Autodesk Inventor part; units mm, degrees
ref_plane "YZ Plane" through (0, 0, 0) normal (1, 0, 0) x (0, 1, 0)
ref_plane "XZ Plane" through (0, 0, 0) normal (0, 1, 0) x (-1, 0, 0)
ref_plane "XY Plane" through (0, 0, 0) normal (0, 0, 1) x (1, 0, 0)
sketch "Sketch1" plane through (0, 0, 0) normal (0, 0, 1) x (1, 0, 0)
  line L0 (-185.0798, 623.3432) -> (284.8202, 623.3432)
  line L1 (284.8202, 623.3432) -> (284.8202, -278.3568)
  line L2 (284.8202, -278.3568) -> (-185.0798, -278.3568)
  line L3 (-185.0798, -278.3568) -> (-185.0798, 623.3432)
  point P0 (0, 0)
  dimension "d0" = 901.7
  dimension "d1" = 469.9
extrude "Board" add sketch "Sketch1" along normal blind 19.05
sketch "Sketch6" plane through (0, 0, 0) normal (0, 0, -1) x (-1, 0, 0)
  line L0 (-284.8202, 483.6432) -> (185.0798, 483.6432)
  line L1 (185.0798, 483.6432) -> (185.0798, 464.5932)
  line L2 (185.0798, 464.5932) -> (-284.8202, 464.5932)
  line L3 (-284.8202, 464.5932) -> (-284.8202, 483.6432)
  line L4 (185.0798, 623.3432) -> (-284.8202, 623.3432)
  line L5 (185.0798, -278.3568) -> (185.0798, 623.3432)
  line L6 (-284.8202, 623.3432) -> (-284.8202, -278.3568)
  line L7 (-284.8202, 29.6182) -> (185.0798, 29.6182)
  line L8 (185.0798, 29.6182) -> (185.0798, 10.5682)
  line L9 (185.0798, 10.5682) -> (-284.8202, 10.5682)
  line L10 (-284.8202, 10.5682) -> (-284.8202, 29.6182)
  point P0 (0, 0)
  dimension "d30" = 19.05
  dimension "d37" = 434.975
  dimension "d119" = 139.7
extrude "Right Shelf Dados" cut sketch "Sketch6" against normal blind 6.35 contours L0 L1 L2 L3 | L7 L5 L9 L6
sketch "Sketch32" plane through (0, 0, 0) normal (0, 0, -1) x (-1, 0, 0)
  line L0 (-157.8202, -78.3318) -> (185.0798, -78.3318)
  line L1 (185.0798, -78.3318) -> (185.0798, -84.6818)
  line L2 (185.0798, -84.6818) -> (-157.8202, -84.6818)
  line L3 (-157.8202, -84.6818) -> (-157.8202, -78.3318)
  line L4 (-157.8202, -173.5818) -> (185.0798, -173.5818)
  line L5 (185.0798, -173.5818) -> (185.0798, -179.9318)
  line L6 (185.0798, -179.9318) -> (-157.8202, -179.9318)
  line L7 (-157.8202, -179.9318) -> (-157.8202, -173.5818)
  line L8 (-284.8202, 623.3432) -> (-284.8202, -278.3568)
  line L9 (185.0798, 623.3432) -> (185.0798, -278.3568)
  line L10 (-284.8202, -278.3568) -> (185.0798, -278.3568)
  point P0 (0, 0)
  point P1 (-284.8202, 10.5682)
  dimension "d142" = 88.9
  dimension "d143" = 6.35
  dimension "d146" = 342.9
  dimension "d167" = 127
  dimension "d170" = 98.425
extrude "Right Wine Rack Horizonal Dados" cut sketch "Sketch32" against normal blind 6.35
sketch "Sketch33" plane through (0, 0, 0) normal (0, 0, -1) x (-1, 0, 0)
  line L0 (185.0798, 10.5682) -> (-284.8202, 10.5682)
  line L1 (70.7798, 10.5682) -> (77.1298, 10.5682)
  line L2 (77.1298, 10.5682) -> (77.1298, -278.3568)
  line L3 (77.1298, -278.3568) -> (70.7798, -278.3568)
  line L4 (70.7798, -278.3568) -> (70.7798, 10.5682)
  line L5 (-157.8202, -84.6818) -> (-157.8202, -78.3318)
  line L6 (-284.8202, -278.3568) -> (185.0798, -278.3568)
  point P0 (0, 0)
  dimension "d149" = 6.35
  dimension "d168" = 228.6
extrude "Right Wine Rack Vertical Dado" cut sketch "Sketch33" against normal blind 6.35
sketch "Sketch7" plane through (0, 0, 19.05) normal (0, 0, 1) x (1, 0, 0)
  line L0 (-185.0798, 483.6432) -> (284.8202, 483.6432)
  line L1 (284.8202, 483.6432) -> (284.8202, 464.5932)
  line L2 (284.8202, 464.5932) -> (-185.0798, 464.5932)
  line L3 (-185.0798, 464.5932) -> (-185.0798, 483.6432)
  line L4 (284.8202, 483.6432) -> (-185.0798, 483.6432)
  line L5 (-185.0798, 464.5932) -> (284.8202, 464.5932)
  line L6 (284.8202, -278.3568) -> (284.8202, 623.3432)
  line L7 (-185.0798, 623.3432) -> (-185.0798, -278.3568)
  line L8 (-185.0798, 29.6182) -> (284.8202, 29.6182)
  line L9 (284.8202, 29.6182) -> (284.8202, 10.5682)
  line L10 (284.8202, 10.5682) -> (-185.0798, 10.5682)
  line L11 (-185.0798, 10.5682) -> (-185.0798, 29.6182)
  point P0 (0, 0)
  point P1 (284.8202, 20.0932)
  dimension "d36" = 434.975
extrude "Left Shelf Dados" cut sketch "Sketch7" against normal blind 6.35 contours L0 L1 L2 L3 | L8 L6 L10 L7
sketch "Sketch34" plane through (0, 0, 19.05) normal (0, 0, 1) x (1, 0, 0)
  line L0 (157.8202, -78.3318) -> (-185.0798, -78.3318)
  line L1 (-185.0798, -78.3318) -> (-185.0798, -84.6818)
  line L2 (-185.0798, -84.6818) -> (157.8202, -84.6818)
  line L3 (157.8202, -84.6818) -> (157.8202, -78.3318)
  line L4 (157.8202, -173.5818) -> (-185.0798, -173.5818)
  line L5 (-185.0798, -173.5818) -> (-185.0798, -179.9318)
  line L6 (-185.0798, -179.9318) -> (157.8202, -179.9318)
  line L7 (157.8202, -179.9318) -> (157.8202, -173.5818)
  line L8 (284.8202, -278.3568) -> (284.8202, 10.5682)
  line L9 (-185.0798, 10.5682) -> (-185.0798, 483.6432)
  line L10 (-185.0798, -278.3568) -> (284.8202, -278.3568)
  point P0 (0, 0)
  dimension "d153" = 6.35
  dimension "d155" = 88.9
  dimension "d164" = 127
  dimension "d171" = 98.425
extrude "Left Wine Rack Horizontal Dados" cut sketch "Sketch34" against normal blind 6.35
sketch "Sketch35" plane through (0, 0, 19.05) normal (0, 0, 1) x (1, 0, 0)
  line L0 (284.8202, 10.5682) -> (-185.0798, 10.5682)
  line L1 (-77.1298, 10.5682) -> (-70.7798, 10.5682)
  line L2 (-70.7798, 10.5682) -> (-70.7798, -278.3568)
  line L3 (-70.7798, -278.3568) -> (-77.1298, -278.3568)
  line L4 (-77.1298, -278.3568) -> (-77.1298, 10.5682)
  line L5 (157.8202, -78.3318) -> (157.8202, -84.6818)
  line L6 (-185.0798, -278.3568) -> (284.8202, -278.3568)
  point P0 (0, 0)
  dimension "d159" = 6.35
  dimension "d165" = 228.6
extrude "Left Wine Rack  Vertical Dado" cut sketch "Sketch35" against normal blind 6.35
sketch "Sketch10" plane through (0, 0, 19.05) normal (0, 0, 1) x (1, 0, 0)
  line L0 (284.8202, -278.3568) -> (-185.0798, -278.3568)
  line L1 (-185.0798, 623.3432) -> (-172.3798, 623.3432)
  line L2 (-172.3798, 623.3432) -> (-172.3798, -278.3568)
  line L3 (-172.3798, -278.3568) -> (-185.0798, -278.3568)
  line L4 (-185.0798, -278.3568) -> (-185.0798, 623.3432)
  point P0 (0, 0)
  point P1 (-77.1298, -278.3568)
  dimension "d48" = 12.7
extrude "Vertical Wire Channel" cut sketch "Sketch10" against normal blind 6.35
sketch "Sketch12" plane through (-185.0798, -278.3568, 12.7) normal (-1, 0, 0) x (0, 0, 1)
  line L0 (-6.35, 742.95) -> (0, 742.95)
  line L1 (0, 742.95) -> (0, 749.3)
  line L2 (0, 749.3) -> (-6.35, 749.3)
  line L3 (-6.35, 749.3) -> (-6.35, 742.95)
  line L4 (0, 0) -> (0, 901.7)
  line L5 (-6.35, 742.95) -> (-12.7, 742.95)
  dimension "d51" = 6.35
extrude "Top Horizontal Wire Channel" cut sketch "Sketch12" against normal blind 12.7
sketch "Sketch20" plane through (0, 0, 0) normal (0, 0, -1) x (-1, 0, 0)
  line L0 (185.0798, 623.3432) -> (-284.8202, 623.3432)
  line L1 (-284.8202, 29.6182) -> (185.0798, 29.6182)
  line L2 (185.0798, 623.3432) -> (178.7298, 623.3432)
  line L3 (178.7298, 623.3432) -> (178.7298, 29.6182)
  line L4 (178.7298, 29.6182) -> (185.0798, 29.6182)
  line L5 (185.0798, 29.6182) -> (185.0798, 623.3432)
  point P0 (0, 0)
  dimension "d99" = 6.35
extrude "Rear Top Panel Dado" cut sketch "Sketch20" against normal blind 12.7
sketch "Sketch21" plane through (-185.0798, -278.3568, 0) normal (-1, 0, 0) x (0, 0, 1)
  line L0 (0, 200.025) -> (0, 288.925)
  line L1 (0, 288.925) -> (6.35, 288.925)
  line L2 (6.35, 288.925) -> (6.35, 0)
  line L3 (0, 0) -> (0, 288.925)
  line L4 (0, 0) -> (6.35, 0)
  line L5 (0, 0) -> (12.7, 0)
extrude "Bottom Panel Dado" cut sketch "Sketch21" against normal blind 6.35
properties part number "Vertical Shelf cut short (2.3.2018)"
Verification items for the finished model (mm, model axes). A direction names the side the tool comes from. Coordinates: 2 decimals unless noted, no trailing zeros. Order: outer loops, then holes, each group sorted by start corner. A loop starts at its lowest first (then second) coordinate and runs counter-clockwise, first axis right, second up.
1. Sectioned sample at A-A, the plane x = 167. Record the cut outline in (y, z).
Results found:
outline: (-278.36, 0) - (10.57, 0) - (10.57, 6.35) - (29.62, 6.35) - (29.62, 0) - (464.59, 0) - (464.59, 6.35) - (483.64, 6.35) - (483.64, 0) - (623.34, 0) - (623.34, 19.05) - (483.64, 19.05) - (483.64, 12.7) - (464.59, 12.7) - (464.59, 19.05) - (29.62, 19.05) - (29.62, 12.7) - (10.57, 12.7) - (10.57, 19.05) - (-278.36, 19.05) - close
2. Set-up check for faces 4 (the face through (56, 474, 6.35)), 5 (the face through (53, 554, 19.05)): record each of +Z, -Z, +X, -X, +Y, -Y from which the full face is reachable in a straight line by a thin tool's end or side.
Results found:
face 4: -Z, +X, -X
face 5: +Z, +X, -X, +Y, -Y
3. Sectioned sample at B-B, the plane y = -218. Record the cut outline in (x, z).
Results found:
outline: (-185.08, 6.35) - (-178.73, 6.35) - (-178.73, 0) - (-77.13, 0) - (-77.13, 6.35) - (-70.78, 6.35) - (-70.78, 0) - (284.82, 0) - (284.82, 19.05) - (-70.78, 19.05) - (-70.78, 12.7) - (-77.13, 12.7) - (-77.13, 19.05) - (-172.38, 19.05) - (-172.38, 12.7) - (-185.08, 12.7) - close
4. Sectioned sample at C-C, the plane y = 202. Record the cut outline in (x, z).
Results found:
outline: (-178.73, 0) - (284.82, 0) - (284.82, 19.05) - (-172.38, 19.05) - (-172.38, 12.7) - (-178.73, 12.7) - close
5. Release check for a two-part mould opening along Y. For faces 1 (the face through (53, -278.357, 9)), 2 (the face through (-56, 12, 12.7)), 3 (the face through (105, -132, 19.05)) record: +Y half, -Y half, draft (parallel to the pull), parting line (faces both ways), or undercut.
Results found:
face 1: -Y half
face 2: undercut
face 3: draft
6. Scan lines: line 1 (Y direction, x = 254.5, z = 4.5); line 2 (Y direction, x = -24, z = 17.25); line 3 (X direction, y = -105, z = 3). Record each from-to range of solid material in increasing order.
Results found:
line 1: y = -278.36 to 10.57, 29.62 to 464.59, 483.64 to 623.34
line 2: y = -278.36 to -179.93, -173.58 to -84.68, -78.33 to 10.57, 29.62 to 464.59, 483.64 to 623.34
line 3: x = -178.73 to -77.13, -70.78 to 284.82
7. Go/stop test with flat-tipped pins: pin 1 Ø3 at (y, z) = (-80.5, 2.5) entering from -X; pin 2 Ø5 at (y, z) = (-12, 2) entering from -X; pin 3 Ø1.9 at (y, z) = (325.5, 16.5) entering from -X. Record where each tip stops, or that it passes through.
Results found:
pin 1: stops at x = 157.82
pin 2: stops at x = -178.73
pin 3: stops at x = -172.38
